For this review, use the dimensioned drawing (mm, ordinates from the lowest corner) and the shaded views. Round coordinates to 2 decimals unless told otherwise and drop trailing zeros. Loops run counter-clockwise (first coordinate to the right, second up) from the corner with the lowest first, then second, coordinate; pieces in that order, holes last. Notation, with made-up numbers: (58, 40.5) - (63, 40.5) arc R21 ccw to (63, 59.5) - close; hole circle Ø11 at (25.5, 72). An arc over 180 degrees is marked (long way). One line per question, with ' | ' between items. Start each with the question number.
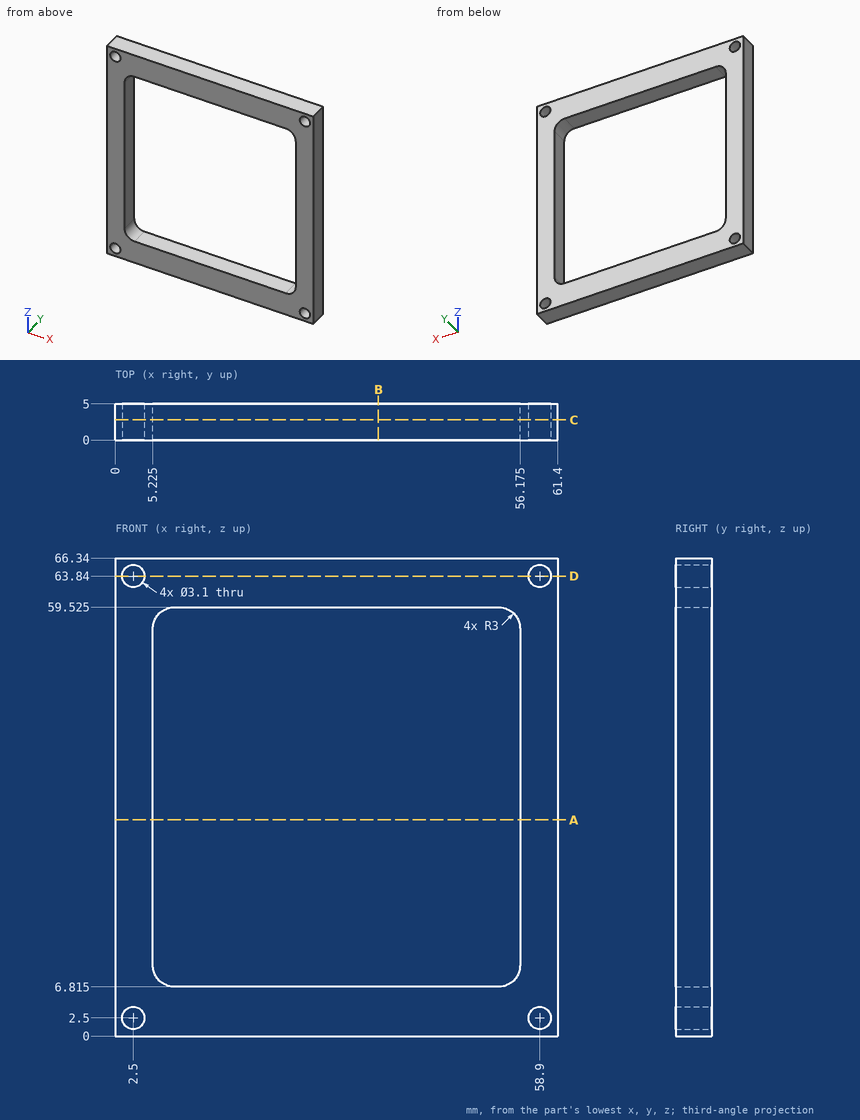
1. Take a section at C-C, the plane y = 2.8. Give the boundary of the cut face in (x, z) (3 decimals).
2. Clearance check with flat-ended pins moving along their axes: P1, Ø2, axis at x = 47, y = 3.5, coming from the -Z side; P2, Ø2.5, axis at x = 58.9, z = 2.5, coming from the -Y side. State where each tip first meets the part, or that it passes through.
3. To check wall thickness, follow line 1 along X through (y, z) = (2.2, 63.84); line 2 along Z through (x, y) = (53, 1.7) (3 decimals); line 3 along X through (y, z) = (0.75, 45.5) (3 decimals). State the ranges of each line that lie inside material, in increasing order.
4. Take a section at A-A, the plane z = 30. Give the boundary of the cut face in (x, y) (3 decimals), then the cut area to 4 significant figures.
5. Take a section at B-B, the plane x = 36.5. Give the boundary of the cut face in (y, z) (3 decimals).
6. Take a section at D-D, the plane z = 63.84. Give the boundary of the cut face in (x, y).
Answer list:
1) outline: (0, 0) - (61.4, 0) - (61.4, 66.34) - (0, 66.34) - close; hole circle Ø3.1 at (2.5, 2.5); hole circle Ø3.1 at (2.5, 63.84); hole (5.225, 9.815) arc R3 ccw to (8.225, 6.815) - (53.175, 6.815) arc R3 ccw to (56.175, 9.815) - (56.175, 56.525) arc R3 ccw to (53.175, 59.525) - (8.225, 59.525) arc R3 ccw to (5.225, 56.525) - close; hole circle Ø3.1 at (58.9, 2.5); hole circle Ø3.1 at (58.9, 63.84)
2) P1: stops at z = 0 | P2: passes through
3) line 1: x = 0 to 0.95, 4.05 to 57.35, 60.45 to 61.4 | line 2: z = 0 to 6.815, 59.525 to 66.34 | line 3: x = 0 to 5.225, 56.175 to 61.4
4) outline: (0, 0) - (5.225, 0) - (5.225, 5) - (0, 5) - close; (56.175, 0) - (61.4, 0) - (61.4, 5) - (56.175, 5) - close | area: 52.25 mm²
5) outline: (0, 0) - (5, 0) - (5, 6.815) - (0, 6.815) - close; (0, 59.525) - (5, 59.525) - (5, 66.34) - (0, 66.34) - close
6) outline: (0, 0) - (0.95, 0) - (0.95, 5) - (0, 5) - close; (4.05, 0) - (57.35, 0) - (57.35, 5) - (4.05, 5) - close; (60.45, 0) - (61.4, 0) - (61.4, 5) - (60.45, 5) - close
